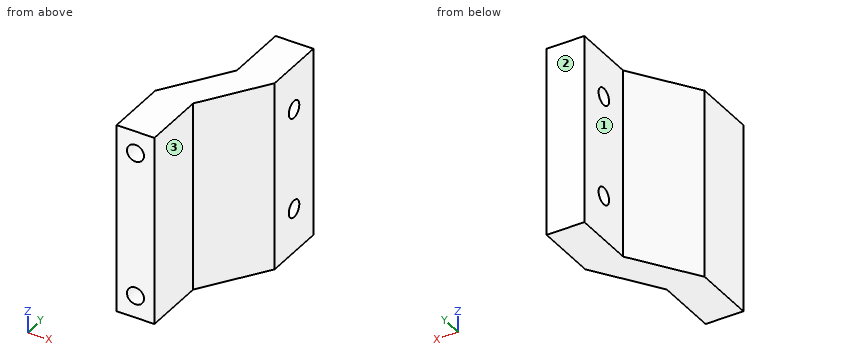
from build123d import *

# Parameters (mm, degrees)
BOSS_EXTRUDE1_DEPTH = 30
SKETCH2_R           = 1.35
CUT_EXTRUDE1_DEPTH  = 8.5
CUT_EXTRUDE2_REACH  = 44.96
SKETCH3_R           = 1.35


with BuildPart() as part:
    # Sketch1 → Boss-Extrude1 (new body)
    with BuildSketch(Plane.XY):
        Polygon((0, 0), (6, 0), (6, 10), (12.75, 20), (12.75, 30), (6.75, 30), (6.75, 20), (0, 10), align=None)
    extrude(amount=BOSS_EXTRUDE1_DEPTH)

    # Sketch2 → Cut-Extrude1 (cut)
    with BuildSketch(Plane.XZ):
        with Locations(Location((3, 26.5, 0), (0, 0, 270))):
            Circle(SKETCH2_R)
        with Locations(Location((3, 3.5, 0), (0, 0, 270))):
            Circle(SKETCH2_R)
    extrude(amount=-CUT_EXTRUDE1_DEPTH, mode=Mode.SUBTRACT)

    # Sketch3 → Cut-Extrude2 (cut, up to next)
    with BuildSketch(Plane.ZY.offset(-6.75), mode=Mode.PRIVATE) as cut_extrude2_sk1:
        with Locations(Location((7, 25, 0), (0, 0, 270))):
            Circle(SKETCH3_R)
    cut_extrude2_tool1 = extrude(cut_extrude2_sk1.sketch, amount=-CUT_EXTRUDE2_REACH, mode=Mode.PRIVATE) & part.part
    # Sketch3 → Cut-Extrude2 (cut, up to next)
    with BuildSketch(Plane.ZY.offset(-6.75), mode=Mode.PRIVATE) as cut_extrude2_sk2:
        with Locations(Location((23, 25, 0), (0, 0, 270))):
            Circle(SKETCH3_R)
    cut_extrude2_tool2 = extrude(cut_extrude2_sk2.sketch, amount=-CUT_EXTRUDE2_REACH, mode=Mode.PRIVATE) & part.part
    add(cut_extrude2_tool1.solids().sort_by_distance((6.75, 25, 7))[0], mode=Mode.SUBTRACT)
    add(cut_extrude2_tool2.solids().sort_by_distance((6.75, 25, 23))[0], mode=Mode.SUBTRACT)


solid = part.part
Design review of the part built by this model. Coordinates are the model's own, in mm. Face numbers are marked on the shaded views. A direction names the side the tool comes from. Give positions to 0.01 mm unless a question says otherwise; leave off trailing zeros. Order: outer loops, then holes, each group sorted by start corner. A loop starts at its lowest first (then second) coordinate and runs counter-clockwise, first axis right, second up.
1. To check wall thickness, follow L1, parallel to Z at x = 9.85, y = 25; L2, parallel to X at y = 2.25, z = 26.5; L3, parallel to X at y = 1.5, z = 8. State the ranges of each line that lie inside material, in increasing order.
Solution:
L1: z = 0 to 5.65, 8.35 to 21.65, 24.35 to 30
L2: x = 0 to 1.65, 4.35 to 6
L3: x = 0 to 6
2. For pin 1 Ø5 at (x, z) = (9, 24.5) entering from -Y; pin 2 Ø1.5 at (x, z) = (7.5, 15.5) entering from -Y; pin 3 Ø8 at (y, z) = (4.5, 9) entering from +X; pin 4 Ø2 at (y, z) = (25, 23) entering from -X, all flat-tipped, find the tip position at first contact; note any pin that passes through.
Solution:
pin 1: stops at y = 10.74
pin 2: stops at y = 11.11
pin 3: stops at x = 6
pin 4: passes through
3. Add section A-A, the plane y = 25. State the section outline as (x, z) points, then the cut area to 3 significant figures.
Solution:
outline: (6.75, 0) - (12.75, 0) - (12.75, 5.65) - (6.75, 5.65) - close; (6.75, 8.35) - (12.75, 8.35) - (12.75, 21.65) - (6.75, 21.65) - close; (6.75, 24.35) - (12.75, 24.35) - (12.75, 30) - (6.75, 30) - close
area: 148 mm2
4. Tool access review of the marked faces 1, 2 and 3: name each direction out of +Z, -Z, +X, -X, +Y, -Y from which nothing blocks a thin tool from reaching the whole face with its end or side.
Solution:
face 1: +Z, -Z, -X, +Y
face 2: +Z, -Z, +X, -X, +Y
face 3: +Z, -Z, +X, -Y
5. Add section D-D, the plane y = 3. State the section outline as (x, z) points.
Solution:
outline: (0, 0) - (6, 0) - (6, 30) - (0, 30) - close; hole circle Ø2.7 at (3, 3.5); hole circle Ø2.7 at (3, 26.5)
6. Add section B-B, the plane z = 3.5. State the section outline as (x, y) points.
Solution:
outline: (0, 0) - (1.65, 0) - (1.65, 8.5) - (4.35, 8.5) - (4.35, 0) - (6, 0) - (6, 10) - (12.75, 20) - (12.75, 30) - (6.75, 30) - (6.75, 20) - (0, 10) - close
7. Add section C-C, the plane x = 9.25. State the section outline as (y, z) points, then the cut area to 3 significant figures.
Solution:
outline: (14.81, 0) - (30, 0) - (30, 30) - (14.81, 30) - close; hole circle Ø2.7 at (25, 7); hole circle Ø2.7 at (25, 23)
area: 444 mm2
